Geometry: final body of the model. Coordinates: model frame, mm. Give positions to 0.01 mm unless a question says otherwise; leave off trailing zeros. Order: outer loops, then holes, each group sorted by start corner. A loop starts at its lowest first (then second) coordinate and runs counter-clockwise, first axis right, second up. Notation, with made-up numbers: (-5.5, 53) - (33.5, 53) arc R32 cw to (33.5, 81) - close; hole circle Ø7 at (15, 14). An arc over 180 degrees is marked (long way). Write item = value, one per line. Start each with the question number.
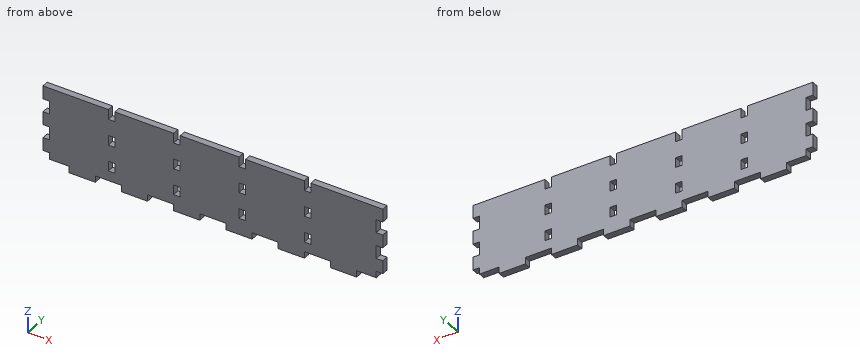
from build123d import *

# Parameters (mm, degrees)
F0_W     = 330.2
F0_H     = 76.2
F1_DEPTH = 6.35
F2_W     = 25.4
F2_H     = 6.35
F2_W_2   = 6.35
F2_H_2   = 12.7
F3_DEPTH = 6.35
F4_W     = 6.35
F4_H     = 9.525
F5_DEPTH = 6.35
F6_W     = 6.35
F6_H     = 6.35
F7_DEPTH = 6.35


# Not quite as in the source:
# - a feature names something its author has since deleted; it is built from what else it names


with BuildPart() as f1:
    # F0 (on Front) → F1 (new body)
    with BuildSketch(Plane.XZ):
        Rectangle(F0_W, F0_H)
    extrude(amount=F1_DEPTH)

    # F2 (on face) → F3 (cut, through all)
    with BuildSketch(Plane.XZ.offset(6.35)):
        with Locations((-152.4, -34.925)):
            Rectangle(F2_W, F2_H)
        with Locations((-101.6, -34.925)):
            Rectangle(F2_W, F2_H)
        with Locations((-50.8, -34.925)):
            Rectangle(F2_W, F2_H)
        with Locations((0, -34.925)):
            Rectangle(F2_W, F2_H)
        with Locations((50.8, -34.925)):
            Rectangle(F2_W, F2_H)
        with Locations((101.6, -34.925)):
            Rectangle(F2_W, F2_H)
        with Locations((152.4, -34.925)):
            Rectangle(F2_W, F2_H)
        with Locations((-161.925, -6.35)):
            Rectangle(F2_W_2, F2_H_2)
        with Locations((-161.925, 19.05)):
            Rectangle(F2_W_2, F2_H_2)
        with Locations((161.925, 19.05)):
            Rectangle(F2_W_2, F2_H_2)
        with Locations((161.925, -6.35)):
            Rectangle(F2_W_2, F2_H_2)
    extrude(amount=-F3_DEPTH, mode=Mode.SUBTRACT)

    # F4 (on face) → F5 (cut, through all)
    with BuildSketch(Plane.XZ.offset(6.35)):
        with Locations((-98.425, 33.3375)):
            Rectangle(F4_W, F4_H)
        with Locations((-98.425, 7.9375)):
            Rectangle(F4_W, F4_H)
        with Locations((-98.425, -17.4625)):
            Rectangle(F4_W, F4_H)
        with Locations((-34.925, 7.9375)):
            Rectangle(F4_W, F4_H)
        with Locations((-34.925, 33.3375)):
            Rectangle(F4_W, F4_H)
        with Locations((-34.925, -17.4625)):
            Rectangle(F4_W, F4_H)
        with Locations((28.575, 7.9375)):
            Rectangle(F4_W, F4_H)
        with Locations((28.575, 33.3375)):
            Rectangle(F4_W, F4_H)
        with Locations((28.575, -17.4625)):
            Rectangle(F4_W, F4_H)
        with Locations((92.075, -17.4625)):
            Rectangle(F4_W, F4_H)
        with Locations((92.075, 7.9375)):
            Rectangle(F4_W, F4_H)
        with Locations((92.075, 33.3375)):
            Rectangle(F4_W, F4_H)
    extrude(amount=-F5_DEPTH, mode=Mode.SUBTRACT)

    # F6 (on face) → F7 (cut, through all)
    with BuildSketch(Plane.XZ.offset(6.35)):
        with Locations((-161.925, -28.575)):
            Rectangle(F6_W, F6_H)
        with Locations((161.925, -28.575)):
            Rectangle(F6_W, F6_H)
    extrude(amount=-F7_DEPTH, mode=Mode.SUBTRACT)


solid = f1.part
Q1. Contact query for flat-ended pins moving along their axis: pin 1 (3 mm diameter, centred on x = 101.5, y = -4.5, fed in from -Z); pin 2 (4 mm diameter, centred on x = -112, z = 23, fed in from +Y); pin 3 (1.9 mm diameter, centred on x = 91, y = -3, fed in from +Z) (3 decimals). Output: stop coordinate, or through.
Q2. Section C-C, the plane x = 4. Return the cut outline in (y, z), then the cut area to 3 significant figures.
Q3. Section B-B, the plane y = -1.5. Count the separate pieces of the cut face and the enclosed holes in it, then the cut area to 3 significant figures.
Q4. Section D-D, the plane z = -6. Return the cut outline in (x, y).
Q5. Section A-A, the plane z = -18. Return the cut outline in (x, y).
Q6. Material intervals for line 1 along X through (y, z) = (-3.5, -14); line 2 along Z through (x, y) = (-101, -1.75) (3 decimals); line 3 along Z through (x, y) = (-38, -0.5) (3 decimals), sorted ascending. Write a range as from..to.
The answers:
q1.pin_1 = -31.75
q1.pin_2 = 0
q1.pin_3 = 28.575
q2.outline = (-6.35, -31.75) - (0, -31.75) - (0, 38.1) - (-6.35, 38.1) - close
q2.area = 444 mm²
q3.separate_pieces = 1
q3.enclosed_holes = 8
q3.area = 22,900 mm²
q4.outline = (-158.75, -6.35) - (158.75, -6.35) - (158.75, 0) - (-158.75, 0) - close
q5.outline = (-165.1, -6.35) - (-101.6, -6.35) - (-101.6, 0) - (-165.1, 0) - close; (-95.25, -6.35) - (-38.1, -6.35) - (-38.1, 0) - (-95.25, 0) - close; (-31.75, -6.35) - (25.4, -6.35) - (25.4, 0) - (-31.75, 0) - close; (31.75, -6.35) - (88.9, -6.35) - (88.9, 0) - (31.75, 0) - close; (95.25, -6.35) - (165.1, -6.35) - (165.1, 0) - (95.25, 0) - close
q6.line_1 = -165.1..-101.6, -95.25..-38.1, -31.75..25.4, 31.75..88.9, 95.25..165.1
q6.line_2 = -31.75..-22.225, -12.7..3.175, 12.7..28.575
q6.line_3 = -38.1..-22.225, -12.7..3.175, 12.7..28.575
